Read the model definition and answer for the solid it produces. Units are mm, in the model's axes. Face numbers are marked on the shaded views. Coordinates: 2 decimals unless noted, no trailing zeros. Order: outer loops, then holes, each group sorted by start corner. A loop starts at its lowest first (then second) coordinate and runs counter-clockwise, first axis right, second up. Notation, with made-up numbers: M -19,16.25 L 37,16.25 A12 cw 37,27.25 Z; hole C 69,-34 d9. An arc over 180 degrees is marked long. Write each question's results on one line, items separated by ' | '.
```python
from build123d import *

# Parameters (mm, degrees)
SKETCH1_R           = 12.7
SKETCH1_R_2         = 9.271
BOSS_EXTRUDE1_DEPTH = 152.4
CHAMFER1_SIZE       = 0.254
FILLET1_R           = 0.254


with BuildPart() as part:
    # Sketch1 → Boss-Extrude1 (new body)
    with BuildSketch(Plane(origin=(0, 0, 0), x_dir=(1, 0, 0), z_dir=(0, 1, 0))):
        with Locations(Location((0, 0, 0), (0, 0, 90))):
            Circle(SKETCH1_R)
        with Locations(Location((0, 0, 0), (0, 0, 90))):
            Circle(SKETCH1_R_2, mode=Mode.SUBTRACT)
    extrude(amount=BOSS_EXTRUDE1_DEPTH)

    # Chamfer1
    chamfer1_edges = [part.edges().sort_by_distance(p)[0] for p in [
        (0, 0, 12.7),
        (0, 152.4, 12.7),
    ]]
    chamfer(chamfer1_edges, length=CHAMFER1_SIZE)

    # Fillet1
    fillet1_edges = [part.edges().sort_by_distance(p)[0] for p in [
        (0, 0, 9.271),
        (0, 152.4, 9.271),
    ]]
    fillet(fillet1_edges, radius=FILLET1_R)


solid = part.part
```
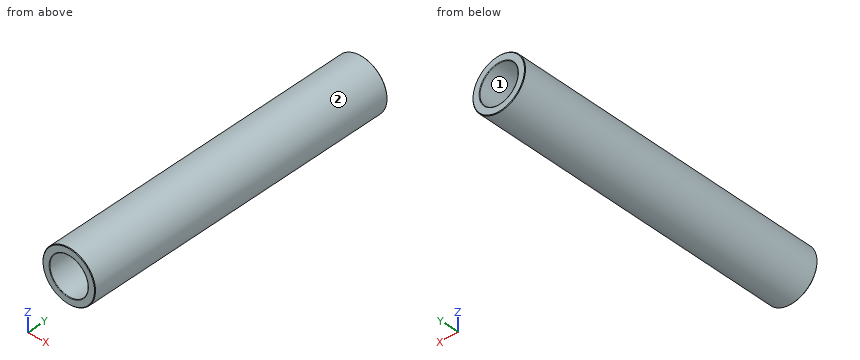
(1) The part is cut by section C-C, the plane y = 118.5. Write down the section's boundary in (x, z).
Conclusion:
outline: C 0,0 d25.4; hole C 0,0 d18.54
(2) The part is cut by section A-A, the plane z = 0. Write down the section's boundary in (x, y) (3 decimals).
Conclusion:
outline: M -12.7,0.254 L -12.446,0 L -9.525,0 A0.254 ccw -9.271,0.254 L -9.271,152.146 A0.254 ccw -9.525,152.4 L -12.446,152.4 L -12.7,152.146 Z; M 9.271,0.254 A0.254 ccw 9.525,0 L 12.446,0 L 12.7,0.254 L 12.7,152.146 L 12.446,152.4 L 9.525,152.4 A0.254 ccw 9.271,152.146 Z
(3) The mould has two halves that part along Z. Classify the marked faces 1 and 2: pulls with the +Z half, pulls with the -Z half, needs draft (parallel to the pull), parting line crosses it, or undercut.
Conclusion:
face 1: undercut | face 2: parting line crosses it
(4) The part is cut by section B-B, the plane x = 0. Write down the section's boundary in (y, z) (3 decimals).
Conclusion:
outline: M 0,-12.446 L 0.254,-12.7 L 152.146,-12.7 L 152.4,-12.446 L 152.4,-9.525 A0.254 ccw 152.146,-9.271 L 0.254,-9.271 A0.254 ccw 0,-9.525 Z; M 0,9.525 A0.254 ccw 0.254,9.271 L 152.146,9.271 A0.254 ccw 152.4,9.525 L 152.4,12.446 L 152.146,12.7 L 0.254,12.7 L 0,12.446 Z
(5) Straight lines are drawn through the part: line 1 (X direction, y = 50, z = 0); line 2 (Z direction, x = -0.75, y = 110); line 3 (Z direction, x = 6.5, y = 63.5). For each, find the intervals that lie inside material, in ascending order.
Conclusion:
line 1: -12.7 to -9.27, 9.27 to 12.7 | line 2: -12.68 to -9.24, 9.24 to 12.68 | line 3: -10.91 to -6.61, 6.61 to 10.91
(6) Given pin 1 (3 mm diameter, centred on x = -5, z = -5.5, fed in from +Y); pin 2 (5 mm diameter, centred on x = 9.5, y = 125, fed in from -Z); pin 3 (1.5 mm diameter, centred on y = 88, z = -4, fed in from +X); pin 4 (8 mm diameter, centred on x = 8, y = 109.5, fed in from -Z), each flat-ended and moving along its own axis, determine where each tip first touches the part or whether it passes through.
Conclusion:
pin 1: through | pin 2: z = -10.6 | pin 3: x = 12.28 | pin 4: z = -12.05
